Input: part model. Units: mm. Frame: model coordinates. Round coordinates to 2 decimals unless told otherwise and drop trailing zeros. Loops run counter-clockwise (first coordinate to the right, second up) from the corner with the lowest first, then second, coordinate; pieces in that order, holes last. Notation, with made-up numbers: (-28.75, 11) -> (2.25, 11) arc R17 cw to (2.25, 22) -> close; hole circle Ø4 at (17.25, 40.5). An arc over 180 degrees is marked (long way). One line per question, with ' | ' between items. Start each with the question number.
Q1. Material intervals for L1, parallel to Y at x = 2.25, z = -3.25; L2, parallel to Z at x = 0.25, y = -2; L3, parallel to Z at x = 4, y = 3, sorted ascending.
Q2. Contact query for flat-ended pins moving along their axis: P1, Ø1, axis at x = -3, y = 11, coming from the -Z side; P2, Ø1, axis at y = -24.5, z = -0.5, coming from the +X side; P3, Ø3, axis at y = 23, z = -2, coming from the +X side. Output: stop coordinate, or through.
Q3. Mould query, pull axis X, two halves, no side actions, for faces 1 (the face through (0, -31.5, -1)), 2 (the face through (0, 27, -3.75)), 3 (the face through (-5.058, -26.43, -4.29)), 4 (the face through (3.142, 26.57, -4.29)). Classes: pulls with the +X half, pulls with the -X half, needs draft (parallel to the pull), parting line crosses it, or undercut.
Q4. Cut plane A-A on x = -0.5. Return loops of the section in (y, z).
Q5. Cut plane C-C on z = 1. Return loops of the section in (x, y), and give its area (3 significant figures).
Q6. Cut plane B-B on y = 5. Return loops of the section in (x, z) (3 decimals).
from build123d import *

# Parameters (mm, degrees)
BOSS_EXTRUDE2_DEPTH     = 31.5
CUT_EXTRUDE1_DEPTH      = 33.294824363
CUT_EXTRUDE1_DEPTH_BACK = 33.294824363
SKETCH2_W               = 2.315915901
SKETCH2_H               = 43
CUT_EXTRUDE2_START      = -21.5
CUT_EXTRUDE2_DEPTH      = 43
FILLET1_R               = 0.3


with BuildPart() as part:
    # Sketch1 → Boss-Extrude2 (new, symmetric)
    with BuildSketch(Plane(origin=(0, 0, 0), x_dir=(1, 0, 0), z_dir=(0, 1, 0))):
        with BuildLine():
            Line((-4.085, -2.5), (4.085, -2.5))
            ThreePointArc((4.085, -2.5), (4.268829006, -2.37878386), (4.229827586, -2.162068966))
            ThreePointArc((4.229827586, -2.162068966), (3.375283995, 0.253722072), (4.608380324, 2.5))
            Line((4.608380324, 2.5), (4.864564522, 3.75))
            Line((4.864564522, 3.75), (5.245248772, 4.815915901))
            Line((5.245248772, 4.815915901), (2.954751228, 4.815915901))
            Line((2.954751228, 4.815915901), (3.335435478, 3.75))
            Line((3.335435478, 3.75), (-3.335435478, 3.75))
            Line((-3.335435478, 3.75), (-2.954751228, 4.815915901))
            Line((-2.954751228, 4.815915901), (-5.245248772, 4.815915901))
            Line((-5.245248772, 4.815915901), (-4.864564522, 3.75))
            Line((-4.864564522, 3.75), (-4.608380324, 2.5))
            ThreePointArc((-4.608380324, 2.5), (-3.375283995, 0.253722072), (-4.229827586, -2.162068966))
            ThreePointArc((-4.229827586, -2.162068966), (-4.268829006, -2.37878386), (-4.085, -2.5))
        make_face()
    extrude(amount=BOSS_EXTRUDE2_DEPTH, both=True)

    # Sketch2 → Cut-Extrude1 (cut, two sides: drawn at the far end of the back side and taken through both)
    with BuildSketch(Plane(origin=(0, 0, 0), x_dir=(0, 0, -1), z_dir=(1, 0, 0)).offset(-CUT_EXTRUDE1_DEPTH_BACK)):
        with Locations((3.657957951, 0)):
            Rectangle(SKETCH2_W, SKETCH2_H)
    extrude(amount=CUT_EXTRUDE1_DEPTH + CUT_EXTRUDE1_DEPTH_BACK, mode=Mode.SUBTRACT)

    # Sketch3 → Cut-Extrude2 (cut)
    with BuildSketch(Plane(origin=(0, 0, 0), x_dir=(1, 0, 0), z_dir=(0, 1, 0)).offset(CUT_EXTRUDE2_START)):
        with BuildLine():
            Line((4.608380324, 2.5), (4.085, 2.5))
            ThreePointArc((4.085, 2.5), (4.268829006, 2.37878386), (4.229827586, 2.162068966))
            ThreePointArc((4.229827586, 2.162068966), (4.412255357, 2.338706331), (4.608380324, 2.5))
        make_face()
        with BuildLine():
            Line((-4.085, 2.5), (-4.608380324, 2.5))
            ThreePointArc((-4.608380324, 2.5), (-4.412255357, 2.338706331), (-4.229827586, 2.162068966))
            ThreePointArc((-4.229827586, 2.162068966), (-4.268829006, 2.37878386), (-4.085, 2.5))
        make_face()
    extrude(amount=CUT_EXTRUDE2_DEPTH, mode=Mode.SUBTRACT)

    # Fillet1
    # the kernel refuses this fillet: 0.3 mm, written as the material it adds along each edge
    with BuildSketch(Plane(origin=(-4.085, 21.5, -2.5), x_dir=(0, 0, -1), z_dir=(1, 0, 0))) as fillet1_piece_1:
        with BuildLine():
            CenterArc((FILLET1_R, -FILLET1_R), FILLET1_R, 90, 90)
            Line((0, -FILLET1_R), (0, 0))
            Line((0, 0), (FILLET1_R, 0))
        make_face()
    extrude(amount=8.17)
    with BuildSketch(Plane(origin=(-4.085, -21.5, -2.5), x_dir=(0, 0, -1), z_dir=(1, 0, 0))) as fillet1_piece_2:
        with BuildLine():
            CenterArc((FILLET1_R, FILLET1_R), FILLET1_R, 180, 90)
            Line((0, FILLET1_R), (0, 0))
            Line((0, 0), (FILLET1_R, 0))
        make_face()
    extrude(amount=8.17)
    with BuildSketch(Plane(origin=(4.085, -21.5, -2.3), x_dir=(0, 0, -1), z_dir=(-1, 0, 0))) as fillet1_piece_3_section:
        with BuildLine():
            CenterArc((0.2 + FILLET1_R, -FILLET1_R), FILLET1_R, 90, 90)
            Line((0.2 + FILLET1_R, 0), (0.2, 0))
            Line((0.2, 0), (0.2, -FILLET1_R))
        make_face()
    fillet1_piece_3 = revolve(axis=Axis((4.085, -21.5, -2.3), (0, -1, 0)), revolution_arc=348.652256653, mode=Mode.PRIVATE)
    fillet1_piece_3 = fillet1_piece_3 - Plane(origin=(6.5, -21.422221686, 0), x_dir=(-0.7241379310344833, 0, 0.6896551724137925), z_dir=(0, 1, 0)) * Cylinder(3.135, 3, mode=Mode.PRIVATE)
    add(fillet1_piece_3)
    with BuildSketch(Plane(origin=(4.085, 21.5, -2.3), x_dir=(0, 0, -1), z_dir=(-1, 0, 0))) as fillet1_piece_4_section:
        with BuildLine():
            CenterArc((0.2 + FILLET1_R, FILLET1_R), FILLET1_R, 180, 90)
            Line((0.2, FILLET1_R), (0.2, 0))
            Line((0.2, 0), (0.2 + FILLET1_R, 0))
        make_face()
    fillet1_piece_4 = revolve(axis=Axis((4.085, 21.5, -2.3), (0, -1, 0)), revolution_arc=348.652256653, mode=Mode.PRIVATE)
    fillet1_piece_4 = fillet1_piece_4 - Plane(origin=(6.5, 21.453136738, 0), x_dir=(-0.7241379310344833, 0, 0.6896551724137925), z_dir=(0, 1, 0)) * Cylinder(3.135, 3, mode=Mode.PRIVATE)
    add(fillet1_piece_4)
    with BuildSketch(Plane(origin=(-4.085, -21.5, -2.3), x_dir=(0.19676320132500988, 0, -0.9804510403912751), z_dir=(-0.9804510403912751, 0, -0.19676320132500988))) as fillet1_piece_5_section:
        with BuildLine():
            CenterArc((-0.2 - FILLET1_R, -FILLET1_R), FILLET1_R, 0, 90)
            Line((-0.2, -FILLET1_R), (-0.2, 0))
            Line((-0.2, 0), (-0.2 - FILLET1_R, 0))
        make_face()
    fillet1_piece_5 = revolve(axis=Axis((-4.085, -21.5, -2.3), (0, -1, 0)), revolution_arc=348.652256653, mode=Mode.PRIVATE)
    fillet1_piece_5 = fillet1_piece_5 - Plane(origin=(-6.5, -21.422220157, 0), x_dir=(0.6033874565748113, 0, -0.7974481658692183), z_dir=(0, 1, 0)) * Cylinder(3.135, 2, mode=Mode.PRIVATE)
    add(fillet1_piece_5)
    with BuildSketch(Plane(origin=(-4.085, 21.5, -2.3), x_dir=(0.1967632013250235, 0, -0.9804510403912723), z_dir=(-0.9804510403912723, 0, -0.1967632013250235))) as fillet1_piece_6_section:
        with BuildLine():
            CenterArc((-0.2 - FILLET1_R, FILLET1_R), FILLET1_R, 270, 90)
            Line((-0.2, FILLET1_R), (-0.2, 0))
            Line((-0.2, 0), (-0.2 - FILLET1_R, 0))
        make_face()
    fillet1_piece_6 = revolve(axis=Axis((-4.085, 21.5, -2.3), (0, -1, 0)), revolution_arc=348.652256653, mode=Mode.PRIVATE)
    fillet1_piece_6 = fillet1_piece_6 - Plane(origin=(-6.5, 21.422220134, 0), x_dir=(0.6033874565748113, 0, -0.7974481658692183), z_dir=(0, 1, 0)) * Cylinder(3.135, 2, mode=Mode.PRIVATE)
    add(fillet1_piece_6)


solid = part.part
Results:
1) L1: -31.5 to -21.5, 21.5 to 31.5 | L2: -2.5 to 2.5 | L3: -2.5 to -1.89, 1.89 to 2.5
2) P1: z = -2.5 | P2: x = 3.53 | P3: x = 4.81
3) face 1: needs draft | face 2: undercut | face 3: pulls with the -X half | face 4: undercut
4) outline: (-31.5, -3.75) -> (-21.5, -3.75) -> (-21.5, -2.8) arc R0.3 cw to (-21.2, -2.5) -> (21.2, -2.5) arc R0.3 cw to (21.5, -2.8) -> (21.5, -3.75) -> (31.5, -3.75) -> (31.5, 2.5) -> (-31.5, 2.5) -> close
5) outline: (-3.53, -31.5) -> (3.53, -31.5) -> (3.53, 31.5) -> (-3.53, 31.5) -> close | area: 445 mm^2
6) outline: (-4.23, -2.162) arc R0.2 ccw to (-4.085, -2.5) -> (4.085, -2.5) arc R0.2 ccw to (4.23, -2.162) arc R3.135 cw to (4.23, 2.162) arc R0.2 ccw to (4.085, 2.5) -> (-4.085, 2.5) arc R0.2 ccw to (-4.23, 2.162) arc R3.135 cw to start
